from build123d import *

# Parameters (mm, degrees)
SKETCH1_W           = 19.05
SKETCH1_H           = 19.05
SKETCH1_W_2         = 15.875
SKETCH1_H_2         = 15.875
BOSS_EXTRUDE1_DEPTH = 379.4633
SHELF_HOLES_REACH   = 21.05
SKETCH2_R           = 2.4257
CUT_EXTRUDE1_REACH  = 21.05
SKETCH3_R           = 4.7625


with BuildPart() as part:
    # Sketch1 → Boss-Extrude1 (new body, symmetric)
    with BuildSketch(Plane.ZX):
        Rectangle(SKETCH1_W, SKETCH1_H)
        Rectangle(SKETCH1_W_2, SKETCH1_H_2, mode=Mode.SUBTRACT)
    extrude(amount=BOSS_EXTRUDE1_DEPTH, both=True)

    # Sketch2 → Shelf Holes (cut, up to next)
    with BuildSketch(Plane.XY.offset(9.525), mode=Mode.PRIVATE) as shelf_holes_sk1:
        with Locations((0, -49.2633)):
            Circle(SKETCH2_R)
    shelf_holes_tool1 = extrude(shelf_holes_sk1.sketch, amount=-SHELF_HOLES_REACH, mode=Mode.PRIVATE) & part.part
    add(shelf_holes_tool1.solids().sort_by_distance((0, -49.2633, 9.525))[0], mode=Mode.SUBTRACT)
    # Sketch2 → Shelf Holes (cut, up to next)
    with BuildSketch(Plane.XY.offset(9.525), mode=Mode.PRIVATE) as shelf_holes_sk2:
        with Locations((0, 230.1367)):
            Circle(SKETCH2_R)
    shelf_holes_tool2 = extrude(shelf_holes_sk2.sketch, amount=-SHELF_HOLES_REACH, mode=Mode.PRIVATE) & part.part
    add(shelf_holes_tool2.solids().sort_by_distance((0, 230.1367, 9.525))[0], mode=Mode.SUBTRACT)

    # Sketch3 → Cut-Extrude1 (cut, up to next)
    with BuildSketch(Plane(origin=(0, 0, -9.525), x_dir=(-1, 0, 0), z_dir=(0, 0, -1)), mode=Mode.PRIVATE) as cut_extrude1_sk1:
        with Locations((0, 112.3823)):
            Circle(SKETCH3_R)
    cut_extrude1_tool1 = extrude(cut_extrude1_sk1.sketch, amount=-CUT_EXTRUDE1_REACH, mode=Mode.PRIVATE) & part.part
    add(cut_extrude1_tool1.solids().sort_by_distance((0, 112.3823, -9.525))[0], mode=Mode.SUBTRACT)
    # Sketch3 → Cut-Extrude1 (cut, up to next)
    with BuildSketch(Plane(origin=(0, 0, -9.525), x_dir=(-1, 0, 0), z_dir=(0, 0, -1)), mode=Mode.PRIVATE) as cut_extrude1_sk2:
        with Locations((0, -115.8621)):
            Circle(SKETCH3_R)
    cut_extrude1_tool2 = extrude(cut_extrude1_sk2.sketch, amount=-CUT_EXTRUDE1_REACH, mode=Mode.PRIVATE) & part.part
    add(cut_extrude1_tool2.solids().sort_by_distance((0, -115.8621, -9.525))[0], mode=Mode.SUBTRACT)


solid = part.part
Can you work these out from the model? Positions are in its coordinate system, mm. A direction names the side the tool comes from. Round coordinates to 2 decimals unless told otherwise and drop trailing zeros. Loops run counter-clockwise (first coordinate to the right, second up) from the corner with the lowest first, then second, coordinate; pieces in that order, holes last. Notation, with made-up numbers: (24, 87) - (54, 87) arc R20 cw to (54, 109) - close; hole circle Ø6 at (5.25, 51.5). An arc over 180 degrees is marked (long way). Answer in a Markdown table with one row per item. Add a question column.
Q1. We'd pull the mould along Z, two halves only. Please class faces 1 (the flat face through (0, 5, 9.525)), 2 (the flat face through (-7.938, 5, 0)), 3 (the flat face through (9.525, 5, 0)): pulls with the +Z half, pulls with the -Z half, needs draft (parallel to the pull), parting line crosses it, or undercut.
Q2. For pin 1 Ø4.5 at (x, y) = (0, -49.26) entering from +Z; pin 2 Ø4 at (x, z) = (7, -6) entering from +Y; pin 3 Ø4 at (x, z) = (-4, 1.5) entering from -Y, each with a flat end and sliding along its axis, tell me the tip position at first contact or that it passes through.
Q3. I want a section at A-A on y = -152.5. List the corners of the cut face in (x, z) for me (1 decimal), and give its area (3 significant figures).
Q4. I need wall thicknesses on L1, parallel to Y at x = 0, z = 8.7; L2, parallel to Z at x = -3, y = 192.5 (1 decimal). Which ranges of each line are inside material? Lowest first, please.
Q5. Which directions (+Z, -Z, +X, -X, +Y, -Y) give clear straight access to the entire face, cutting with the end or side of a thin tool? Please do faces 4 (the flat face through (0, 5, -7.938)), 5 (the flat face through (0, 5, -9.525)).
Q6. I want a section at B-B on z = -4.5. List the corners of the cut face in (x, y) for me (1 decimal), and give its area (3 significant figures).
A:
| question | item | result |
|---|---|---|
| 1 | face 1 | pulls with the +Z half |
| 1 | face 2 | undercut |
| 1 | face 3 | needs draft |
| 2 | pin 1 | z = -7.94 |
| 2 | pin 2 | y = 379.46 |
| 2 | pin 3 | through |
| 3 | outline | (-9.5, -9.5) - (9.5, -9.5) - (9.5, 9.5) - (-9.5, 9.5) - close; hole (-7.9, -7.9) - (7.9, -7.9) - (7.9, 7.9) - (-7.9, 7.9) - close |
| 3 | area | 111 mm^2 |
| 4 | L1 | -379.46 to -51.69, -46.84 to 227.71, 232.56 to 379.46 |
| 4 | L2 | -9.5 to -7.9, 7.9 to 9.5 |
| 5 | face 4 | +Y, -Y |
| 5 | face 5 | -Z, +X, -X, +Y, -Y |
| 6 | outline | (-9.5, -379.5) - (-7.9, -379.5) - (-7.9, 379.5) - (-9.5, 379.5) - close; (7.9, -379.5) - (9.5, -379.5) - (9.5, 379.5) - (7.9, 379.5) - close |
| 6 | area | 2,410 mm^2 |
